```python
from build123d import *

# Parameters (mm, degrees)
SKETCH3_R           = 10
BOSS_EXTRUDE1_DEPTH = 15


with BuildPart() as part:
    # Sketch2 → Revolve1 (revolve)
    with BuildSketch(Plane.XY):
        Polygon((-195, 0), (195, 0), (195, 44.5), (-175, 44.5), (-175, 54.5), (-195, 54.5), align=None)
    revolve(axis=Axis((-195, 0, 0), (1, 0, 0)))

    # Sketch3 → Boss-Extrude1 (add)
    with BuildSketch(Plane.XY.offset(7.5)):
        with BuildLine():
            Line((195, 22.5), (230, 22.5))
            ThreePointArc((230, 22.5), (252.5, 0), (230, -22.5))
            Line((230, -22.5), (195, -22.5))
            Line((195, -22.5), (195, 22.5))
        make_face()
        with Locations((230, 0)):
            Circle(SKETCH3_R, mode=Mode.SUBTRACT)
    boss_extrude1 = extrude(amount=BOSS_EXTRUDE1_DEPTH)

    # Mirror1: Boss-Extrude1 across plane
    add(boss_extrude1.mirror(Plane.XY))


solid = part.part
```
Here's how the part is built. I have some questions about the finished solid (model axes, mm). A direction names the side the tool comes from. Round coordinates to 2 decimals unless told otherwise and drop trailing zeros. Order: outer loops, then holes, each group sorted by start corner. A loop starts at its lowest first (then second) coordinate and runs counter-clockwise, first axis right, second up. Notation, with made-up numbers: M 22,47.5 L 45,47.5 A36 ccw 45,86.5 Z; hole C 88,26 d8. An arc over 180 degrees is marked long. Answer in a Markdown table with one row per item.
Item 1: I'm going to push flat-ended pins straight in: pin 1 (22.5 mm diameter, centred on x = 217, y = 1, fed in from -Z); pin 2 (8 mm diameter, centred on x = 155.5, y = 17.5, fed in from +Z); pin 3 (16.5 mm diameter, centred on x = 216.5, z = 15, fed in from -Y). Where does each tip first touch, or does it pass through?
A:
| item | result |
|---|---|
| pin 1 | stops at z = -22.5 |
| pin 2 | stops at z = 42.4 |
| pin 3 | stops at y = -22.5 |
Item 2: For faces 5 (the face through (213, -22.5, -15)), 6 (the face through (7.41, -32.798, 30.075)), 7 (the face through (212, 22.5, 15)), 8 (the face through (218, 0, -22.5)), which set-ups out of +Z, -Z, +X, -X, +Y, -Y let a thin tool reach every point of the face, with its end or its side?
A:
| item | result |
|---|---|
| face 5 | +Z, -Z, +X, -Y |
| face 6 | +X |
| face 7 | +Z, -Z, +X, +Y |
| face 8 | -Z, +X, +Y, -Y |
Item 3: Imagine slicing it at B-B, the plane z = 0. Write out the boundary of the cut face in (x, y), and give its area (3 significant figures).
A:
| item | result |
|---|---|
| outline | M -195,-54.5 L -175,-54.5 L -175,-44.5 L 195,-44.5 L 195,44.5 L -175,44.5 L -175,54.5 L -195,54.5 Z |
| area | 35,100 mm2 |
Item 4: If I drill on L1, parallel to Y at x = 230, z = 13.75; L2, parallel to Z at x = 218, y = -11; L3, parallel to X at y = -10, z = 32, over which ranges is the centre line in solid material (lowest first)? Write a range as from..to.
A:
| item | result |
|---|---|
| L1 | y = -22.5..-10, 10..22.5 |
| L2 | z = -22.5..-7.5, 7.5..22.5 |
| L3 | x = -195..195 |
Item 5: Thinking about a two-plate mould opening in Z: for faces 1 (the face through (218, 0, 22.5)), 2 (the face through (218, 0, -7.5)), 3 (the face through (218, 0, 7.5)), 4 (the face through (-175, 45, 0)), which applies, +Z half, -Z half, draft (parallel to the pull), parting line (faces both ways), or undercut?
A:
| item | result |
|---|---|
| face 1 | +Z half |
| face 2 | undercut |
| face 3 | undercut |
| face 4 | draft |
Item 6: Imagine slicing it at C-C, the plane y = 17.5. Write out the boundary of the cut face in (x, z).
A:
| item | result |
|---|---|
| outline | M -195,-51.61 L -175,-51.61 L -175,-40.91 L 195,-40.91 L 195,-22.5 L 244.14,-22.5 L 244.14,-7.5 L 195,-7.5 L 195,7.5 L 244.14,7.5 L 244.14,22.5 L 195,22.5 L 195,40.91 L -175,40.91 L -175,51.61 L -195,51.61 Z |
Item 7: Imagine slicing it at A-A, the plane y = 0. Write out the boundary of the cut face in (x, z).
A:
| item | result |
|---|---|
| outline | M -195,-54.5 L -175,-54.5 L -175,-44.5 L 195,-44.5 L 195,-22.5 L 220,-22.5 L 220,-7.5 L 195,-7.5 L 195,7.5 L 220,7.5 L 220,22.5 L 195,22.5 L 195,44.5 L -175,44.5 L -175,54.5 L -195,54.5 Z; M 240,-22.5 L 252.5,-22.5 L 252.5,-7.5 L 240,-7.5 Z; M 240,7.5 L 252.5,7.5 L 252.5,22.5 L 240,22.5 Z |
Item 8: Imagine slicing it at D-D, the plane x = -36. Write out the boundary of the cut face in (y, z), and give its area (3 significant figures).
A:
| item | result |
|---|---|
| outline | C 0,0 d89 |
| area | 6,220 mm2 |
